Could you check a few things on this model? Use its own coordinates, in mm. Face numbers are marked on the shaded views. Coordinates: 2 decimals unless noted, no trailing zeros. Loops run counter-clockwise (first coordinate to the right, second up) from the corner with the lowest first, then second, coordinate; pieces in that order, holes last. Notation, with made-up numbers: (65.5, -7.5) - (100.5, -7.5) arc R30 ccw to (100.5, 27.5) - close; hole circle Ø2 at (15.25, 11.25). An arc over 180 degrees is marked (long way). Use CSV: the item, a comma, the result in double quotes.
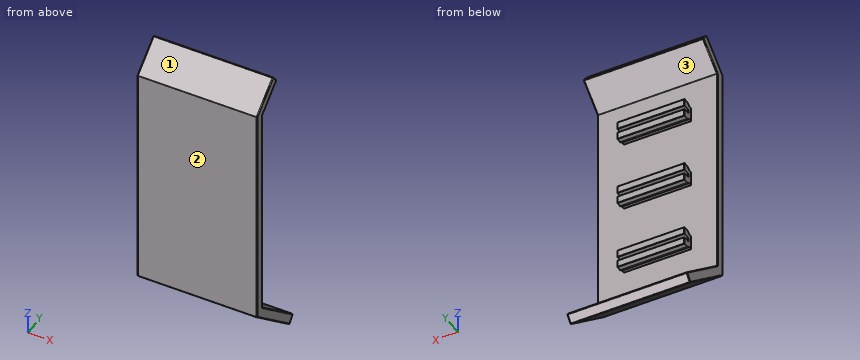
from build123d import *

# Parameters (mm, degrees)
EXTRUDE_1_DEPTH        = 25
EXTRUDE_START          = -5.5
EXTRUDE_2_DEPTH        = 14
PATTERN_LINEAR_1_COUNT = 3
PATTERN_LINEAR_1_PITCH = 15
FILLET_1_R             = 0.1
FILLET_2_R             = 0.2


with BuildPart() as part:
    # 草图1 → 凸台-拉伸1 (new body)
    with BuildSketch(Plane(origin=(0, 0, 0), x_dir=(0, 0, -1), z_dir=(1, 0, 0))):
        Polygon((0, 0), (-7.5, 0), (-11.999513268, 5.362311102), (-13.531602154, 4.076735882), (-8.432615316, -2), (0, -2), (38.432615316, -2), (48.673903032, 10.205091427), (47.141814145, 11.490666647), (37.5, 0), align=None)
    extrude(amount=EXTRUDE_1_DEPTH)

    # 草图2 → 凸台-拉伸2 (add)
    with BuildSketch(Plane(origin=(25, 0, 0), x_dir=(0, 0, -1), z_dir=(1, 0, 0)).offset(EXTRUDE_START)):
        with BuildLine():
            Line((1.5, 0), (-1.5, 0))
            Line((-1.5, 0), (-1.5, 0.677124344))
            ThreePointArc((-1.5, 0.677124344), (-1.780042303, 1.088161527), (-1.95, 1.555590279))
            Line((-1.95, 1.555590279), (-1.95, 2.5))
            Line((-1.95, 2.5), (-0.4, 2.5))
            Line((-0.4, 2.5), (-0.4, 1))
            Line((-0.4, 1), (0.4, 1))
            Line((0.4, 1), (0.4, 2.5))
            Line((0.4, 2.5), (1.95, 2.5))
            Line((1.95, 2.5), (1.95, 1.555590279))
            ThreePointArc((1.95, 1.555590279), (1.780042303, 1.088161527), (1.5, 0.677124344))
            Line((1.5, 0.677124344), (1.5, 0))
        make_face()
    extrude_2 = extrude(amount=-EXTRUDE_2_DEPTH)

    # 阵列(线性)1: 凸台-拉伸2 ×3
    with Locations(*[(0, 0, -i * PATTERN_LINEAR_1_PITCH) for i in range(1, PATTERN_LINEAR_1_COUNT)]):
        add(extrude_2)

    # 圆角1
    fillet_1_edges = [part.edges().sort_by_distance(p)[0] for p in [
        (12.5, 2.5, 0.4),
        (5.5, 2.5, -1.175),
        (12.5, 2.5, -0.4),
        (12.5, 2.5, -1.95),
        (5.5, 2.5, 1.175),
        (12.5, 2.5, 1.95),
        (19.5, 2.5, 1.175),
        (19.5, 2.5, -1.175),
        (12.5, 2.5, -14.6),
        (5.5, 2.5, -16.175),
        (12.5, 2.5, -15.4),
        (12.5, 2.5, -16.95),
        (5.5, 2.5, -13.825),
        (12.5, 2.5, -13.05),
        (19.5, 2.5, -13.825),
        (19.5, 2.5, -16.175),
        (12.5, 2.5, -29.6),
        (5.5, 2.5, -31.175),
        (12.5, 2.5, -30.4),
        (12.5, 2.5, -31.95),
        (5.5, 2.5, -28.825),
        (12.5, 2.5, -28.05),
        (19.5, 2.5, -28.825),
        (19.5, 2.5, -31.175),
    ]]
    fillet(fillet_1_edges, radius=FILLET_1_R)

    # 圆角2
    fillet_2_edges = [part.edges().sort_by_distance(p)[0] for p in [
        (25, 2.681155551, 9.749756634),
        (0, 4.102545714, -43.553259174),
        (0, -2, -15),
        (0, 1.038367941, 10.982108735),
        (0, 4.719523492, 12.765557711),
        (0, 2.681155551, 9.749756634),
        (0, 0, -15),
        (25, 4.719523492, 12.765557711),
        (25, 1.038367941, 10.982108735),
        (12.5, 0, -37.5),
        (12.5, 11.490666647, -47.141814145),
        (12.5, 10.205091427, -48.673903032),
        (12.5, -2, -38.432615316),
        (12.5, -2, 8.432615316),
        (12.5, 4.076735882, 13.531602154),
        (12.5, 5.362311102, 11.999513268),
        (12.5, 0, 7.5),
        (25, -2, -15),
        (25, 4.102545714, -43.553259174),
        (25, 10.847879037, -47.907858588),
        (25, 5.745333323, -42.320907073),
        (25, 0, -15),
        (0, 5.745333323, -42.320907073),
        (0, 10.847879037, -47.907858588),
    ]]
    fillet(fillet_2_edges, radius=FILLET_2_R)


solid = part.part
(1) Suppose I cut it at A-A (z = -5.5). Write out the boundary of the cut face in (x, y), plus the area to 3 significant figures.
Computed:
outline,"(0, -1.8) arc R0.2 ccw to (0.2, -2) - (24.8, -2) arc R0.2 ccw to (25, -1.8) - (25, -0.2) arc R0.2 ccw to (24.8, 0) - (0.2, 0) arc R0.2 ccw to (0, -0.2) - close"
area,"50.0 mm²"
(2) Will these pins go through, and if not, where does the flat tip stop? pin 1 (2 mm diameter, centred on x = 6, y = 5.5, fed in from +Z); pin 2 (1.2 mm diameter, centred on y = 1.5, z = -1, fed in from -X); pin 3 (0.9 mm diameter, centred on x = 9.5, y = 2, fed in from -Z); pin 4 (8 mm diameter, centred on y = 0.5, z = -27, fed in from +X).
Computed:
pin 1,"stops at z = 13.03"
pin 2,"stops at x = 5.5"
pin 3,"stops at z = -42.17"
pin 4,"stops at x = 25"
(3) Thinking about a two-plate mould opening in Z: for the marked faces 1, 2 and 3, which applies, +Z half, -Z half, draft (parallel to the pull), parting line (faces both ways), or undercut?
Computed:
face 1,"+Z half"
face 2,"draft"
face 3,"undercut"
(4) Please list where these lines run through material, in increasing order: line 1 (Y direction, x = 23.75, z = -35); line 2 (Y direction, x = 8.75, z = 0); line 3 (Z direction, x = 15.25, y = 2.75).
Computed:
line 1,"y = -2 to 0"
line 2,"y = -2 to 1"
line 3,"z = -42.42 to -39.81, 9.81 to 12.42"
